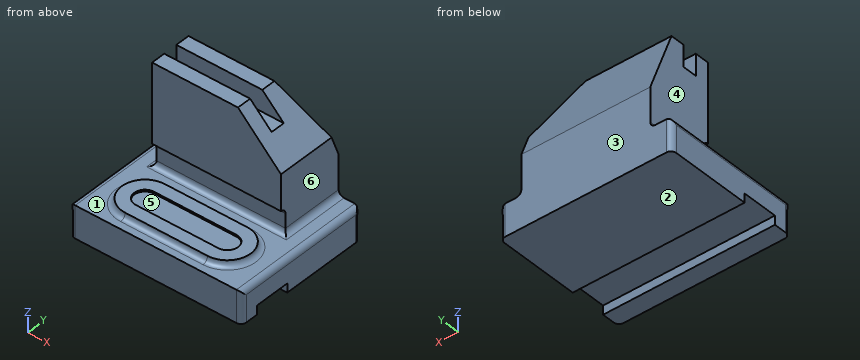
```python
from build123d import *

# Parameters (mm, degrees)
F0_W      = 96
F0_H      = 78
F1_DEPTH  = 18
F3_W      = 72
F3_H      = 38
F5_DEPTH  = 58
F7_DEPTH  = 38
F8_W      = 8
F8_H      = 12
F9_DEPTH  = 60.001
F11_DEPTH = 72.001
F12_W     = 20
F12_H     = 5
F13_DEPTH = 96.001
F14_W     = 46
F14_H     = 26
F15_DEPTH = 3
F16_W     = 46
F16_H     = 12
F17_DEPTH = 1
F18_W     = 3
F18_H     = 14
F19_DEPTH = 72
F20_R     = 2.99999


# Not quite as in the source:
# - a fillet or chamfer is up to 0.001 mm smaller than in the source, because OpenCascade refuses the exact size


with BuildPart() as f1:
    # F0 (on Top) → F1 (new body)
    with BuildSketch(Plane.XY):
        with Locations((48, 39)):
            Rectangle(F0_W, F0_H)
    extrude(amount=F1_DEPTH)

    # F3 (on face) → F5 (join, through all)
    with BuildSketch(Plane.XY.offset(18)):
        with Locations((48, 59)):
            Rectangle(F3_W, F3_H)
    extrude(amount=F5_DEPTH)

    # F6 (on face) → F7 (cut, through all)
    with BuildSketch(Plane.XZ.offset(-40)):
        Polygon((84, 76), (60, 76), (84, 52), align=None)
    extrude(amount=-F7_DEPTH, mode=Mode.SUBTRACT)

    # F8 (on face) → F9 (cut, through all)
    with BuildSketch(Plane(origin=(12, 0, 0), x_dir=(0, -1, 0), z_dir=(-1, 0, 0))):
        with Locations((-52, 70)):
            Rectangle(F8_W, F8_H)
    extrude(amount=-F9_DEPTH, mode=Mode.SUBTRACT)

    # F10 (on face) → F11 (cut, through all)
    with BuildSketch(Plane(origin=(12, 0, 0), x_dir=(0, -1, 0), z_dir=(-1, 0, 0))):
        Polygon((-64, 76), (-78, 76), (-78, 40), align=None)
    extrude(amount=-F11_DEPTH, mode=Mode.SUBTRACT)

    # F12 (on face) → F13 (cut, through all)
    with BuildSketch(Plane.YZ.offset(96)):
        with Locations((20, 2.5)):
            Rectangle(F12_W, F12_H)
    extrude(amount=-F13_DEPTH, mode=Mode.SUBTRACT)

    # F14 (on face) → F15 (join)
    with BuildSketch(Plane.XY.offset(18)):
        with Locations((48, 19.9999999999)):
            Rectangle(F14_W, F14_H)
        with BuildLine():
            Line((25, 6.9999999999), (25, 32.9999999999))
            ThreePointArc((25, 32.9999999999), (12, 19.9999999999), (25, 6.9999999999))
        make_face()
        with BuildLine():
            ThreePointArc((71, 6.9999999999), (84, 19.9999999999), (71, 32.9999999999))
            Line((71, 32.9999999999), (71, 6.9999999999))
        make_face()
    extrude(amount=F15_DEPTH)

    # F16 (on face) → F17 (cut, through all)
    with BuildSketch(Plane.XY.offset(21)):
        with Locations((48, 19.9999999999)):
            Rectangle(F16_W, F16_H)
        with BuildLine():
            Line((25, 13.9999999999), (25, 25.9999999999))
            ThreePointArc((25, 25.9999999999), (19, 19.9999999999), (25, 13.9999999999))
        make_face()
        with BuildLine():
            ThreePointArc((71, 13.9999999999), (77, 19.9999999999), (71, 25.9999999999))
            Line((71, 25.9999999999), (71, 13.9999999999))
        make_face()
    extrude(amount=-F17_DEPTH, mode=Mode.SUBTRACT)

    # F18 (on face) → F19 (cut, through all)
    with BuildSketch(Plane.YZ.offset(84)):
        with Locations((41.5, 25)):
            Rectangle(F18_W, F18_H)
    extrude(amount=-F19_DEPTH, mode=Mode.SUBTRACT)

    # F20 (radius 3 in the source; OpenCascade refuses exactly that, so slightly less here)
    f20_edges = [f1.edges().sort_by_distance(p)[0] for p in [
        (48, 43, 32),
        (48, 43, 18),
        (48, 33, 18),
        (48, 7, 18),
        (96, 39, 18),
        (0, 39, 18),
        (84, 60.5, 18),
        (12, 60.5, 18),
        (96, 0, 9),
        (0, 0, 9),
        (0, 78, 9),
        (96, 78, 9),
    ]]
    fillet(f20_edges, radius=F20_R)


solid = f1.part
```
CAD build for the part. Positions are in the model's coordinates, mm. Face numbers are marked on the shaded views. A direction names the side the tool comes from. Round coordinates to 2 decimals unless told otherwise and drop trailing zeros. Write each loop counter-clockwise with the first axis right and the second up, starting at its lowest first coordinate (ties: lowest second). Pieces come first, ordered by that corner, then holes.
Item 1: Tool access for the marked faces 4, 5 and 6: list every direction of +Z, -Z, +X, -X, +Y, -Y with a clear straight run to the whole face (end or side of a thin tool).
Filled in:
face 4: +Z, -X, +Y, -Y
face 5: +Z
face 6: +Z, +X, +Y, -Y
Item 2: Band-saw the part on A-A on y = 54. Write the cut outline in (x, z).
Filled in:
outline: (0, 0) - (96, 0) - (96, 15) arc R3 ccw to (93, 18) - (87, 18) arc R3 cw to (84, 21) - (84, 52) - (72, 64) - (12, 64) - (12, 21) arc R3 cw to (9, 18) - (3, 18) arc R3 ccw to (0, 15) - close
Item 3: Band-saw the part on B-B on z = 49. Write the cut outline in (x, y).
Filled in:
outline: (12, 40) - (84, 40) - (84, 74.5) - (12, 74.5) - close
Item 4: Drop flat-ended pins along their axis: pin 1 Ø13 at (x, z) = (49.5, 68) entering from -Y; pin 2 Ø1.5 at (x, y) = (71.5, 46) entering from +Z; pin 3 Ø9.5 at (x, z) = (49.5, 68) entering from +Y. Give the stop position or say it passes through.
Filled in:
pin 1: stops at y = 40
pin 2: stops at z = 65.25
pin 3: stops at y = 68.96
Item 5: Band-saw the part on D-D on z = 36.5. Write the cut outline in (x, y).
Filled in:
outline: (12, 40) - (84, 40) - (84, 78) - (12, 78) - close
Item 6: Mould opens along Y. For the marked faces 1, 2 and 3 say: released by +Y, released by -Y, zero draft, split by the parting line, or undercut.
Filled in:
face 1: undercut
face 2: zero draft
face 3: released by +Y
Item 7: Band-saw the part on C-C on y = 67. Write the cut outline in (x, z).
Filled in:
outline: (0, 0) - (96, 0) - (96, 15) arc R3 ccw to (93, 18) - (87, 18) arc R3 cw to (84, 21) - (84, 52) - (67.71, 68.29) - (12, 68.29) - (12, 21) arc R3 cw to (9, 18) - (3, 18) arc R3 ccw to (0, 15) - close
Item 8: Drill centre lines: L1, parallel to Y at x = 66.5, z = 4.5; L2, parallel to Z at x = 90.5, y = 57; L3, parallel to Z at x = 40, y = 16.5. Where is each one in solid material? Low to high.
Filled in:
L1: y = 0 to 10, 30 to 78
L2: z = 0 to 18
L3: z = 5 to 20
